Could you check a few things on this model? Use its own coordinates, in mm. A direction names the side the tool comes from. Coordinates: 2 decimals unless noted, no trailing zeros. Answer as CSV lines item,"result". Start each with the question number.
Item 1: We'd pull the mould along Y, two halves only. Please class faces 4 (the flat face through (-12, 9.525, -150)), 5 (the flat face through (12, -9.525, -150)), 6 (the cylindrical face through (15.874, -2.176, -150.266)): +Y half, -Y half, draft (parallel to the pull), parting line (faces both ways), or undercut.
Item 2: On a 3-axis mill with a long thin cutter (end or side, diameter ignored), from which of +Z, -Z, +X, -X, +Y, -Y can I reach the whole of each face in a straight line? I mean faces 1 (the flat face through (19.05, 0, -150)), 2 (the flat face through (11.892, 5, -150)), 3 (the flat face through (0, -2.667, -150)). Say none if no direction works.
Item 3: Suppose I cut it at A-A, the plane z = -233.5. State how many separate pieces and enclosed holes the cut face has, and give its area (3 significant figures).
Item 4: I'm going to push a flat-ended pin straight in: P1, Ø1, axis at y = 7.5, z = -153.5, coming from the +X side. Where does the tip first touch, or does it pass through?
Item 5: If I drill on line 1 along Y through (x, z) = (12.7, -233.5) (3 decimals); line 2 along X through (y, z) = (-3.25, -45); line 3 along X through (y, z) = (3, -258.5), over which ranges is the centre line in solid material (lowest first)? Write a range as [from, to].
Autodesk Inventor part; units mm, degrees
ref_plane "YZ Plane" through (0, 0, 0) normal (1, 0, 0) x (0, 1, 0)
ref_plane "XZ Plane" through (0, 0, 0) normal (0, 1, 0) x (-1, 0, 0)
ref_plane "XY Plane" through (0, 0, 0) normal (0, 0, 1) x (1, 0, 0)
sketch "Sketch1" plane through (0, 0, 0) normal (0, 0, 1) x (1, 0, 0)
  circle A0 centre (12.7, -3.175) radius 3.3274
  arc A1 (-12.1461, 2.3151) -> (-11.8921, 2.5691) centre (-12.1461, 2.5691) ccw
  line L0 (-17.0229, 2.3151) -> (-12.1461, 2.3151)
  arc A2 (-17.2769, 2.5691) -> (-17.0229, 2.3151) centre (-17.0229, 2.5691) ccw
  line L1 (-17.2769, 4.9059) -> (-17.2769, 2.5691)
  arc A3 (-14.4829, 7.6999) -> (-17.2769, 4.9059) centre (-14.4829, 4.9059) ccw
  line L2 (-12.1461, 7.6999) -> (-14.4829, 7.6999)
  arc A4 (-11.8921, 7.4459) -> (-12.1461, 7.6999) centre (-12.1461, 7.4459) ccw
  line L3 (-11.8921, 2.5691) -> (-11.8921, 7.4459)
  circle A5 centre (-12.7, -3.175) radius 3.3274
  arc A6 (12.1461, 7.6999) -> (11.8921, 7.4459) centre (12.1461, 7.4459) ccw
  line L4 (14.4829, 7.6999) -> (12.1461, 7.6999)
  arc A7 (17.2769, 4.9059) -> (14.4829, 7.6999) centre (14.4829, 4.9059) ccw
  line L5 (17.2769, 2.5691) -> (17.2769, 4.9059)
  arc A8 (17.0229, 2.3151) -> (17.2769, 2.5691) centre (17.0229, 2.5691) ccw
  line L6 (12.1461, 2.3151) -> (17.0229, 2.3151)
  arc A9 (11.8921, 2.5691) -> (12.1461, 2.3151) centre (12.1461, 2.5691) ccw
  line L7 (11.8921, 7.4459) -> (11.8921, 2.5691)
  line L8 (-9.4427, 9.525) -> (-14.0829, 9.525)
  arc A10 (-15.6028, 9.525) -> (-14.0829, 9.525) centre (-14.8428, 9.525) ccw
  line L9 (-15.6028, 9.525) -> (-15.875, 9.525)
  arc A11 (-15.875, 9.525) -> (-19.05, 6.35) centre (-15.875, 6.35) ccw
  line L10 (-19.05, 6.35) -> (-19.05, -6.35)
  arc A12 (-19.05, -6.35) -> (-15.875, -9.525) centre (-15.875, -6.35) ccw
  line L11 (-15.875, -9.525) -> (-15.6028, -9.525)
  arc A13 (-14.0829, -9.525) -> (-15.6028, -9.525) centre (-14.8428, -9.525) ccw
  line L12 (-14.0829, -9.525) -> (-9.4578, -9.525)
  arc A14 (-7.9379, -9.525) -> (-9.4578, -9.525) centre (-8.6979, -9.525) ccw
  line L13 (-7.9379, -9.525) -> (7.9379, -9.525)
  arc A15 (9.4578, -9.525) -> (7.9379, -9.525) centre (8.6979, -9.525) ccw
  line L14 (9.4578, -9.525) -> (14.0829, -9.525)
  arc A16 (15.6028, -9.525) -> (14.0829, -9.525) centre (14.8428, -9.525) ccw
  line L15 (15.6028, -9.525) -> (15.875, -9.525)
  arc A17 (15.875, -9.525) -> (19.05, -6.35) centre (15.875, -6.35) ccw
  line L16 (19.05, -6.35) -> (19.05, 6.35)
  arc A18 (19.05, 6.35) -> (15.875, 9.525) centre (15.875, 6.35) ccw
  line L17 (15.875, 9.525) -> (15.6028, 9.525)
  arc A19 (14.0829, 9.525) -> (15.6028, 9.525) centre (14.8428, 9.525) ccw
  line L18 (14.0829, 9.525) -> (9.4427, 9.525)
  arc A20 (7.9228, 9.525) -> (9.4427, 9.525) centre (8.6828, 9.525) ccw
  line L19 (7.9228, 9.525) -> (5.6388, 9.525)
  arc A21 (5.6388, 9.525) -> (4.064, 7.9502) centre (5.6388, 7.9502) ccw
  line L20 (4.064, 7.9502) -> (4.064, 7.0358)
  arc A22 (4.064, 7.0358) -> (5.6388, 5.461) centre (5.6388, 7.0358) ccw
  line L21 (5.6388, 5.461) -> (6.6706, 5.461)
  arc A23 (6.6706, 5.461) -> (6.9246, 5.715) centre (6.6706, 5.715) ccw
  line L22 (6.9246, 5.715) -> (6.9246, 6.081)
  arc A24 (7.1786, 6.335) -> (6.9246, 6.081) centre (7.1786, 6.081) ccw
  line L23 (7.1786, 6.335) -> (9.017, 6.335)
  arc A25 (10.287, 5.065) -> (9.017, 6.335) centre (9.017, 5.065) ccw
  line L24 (10.287, 5.065) -> (10.287, 3.6128)
  arc A26 (10.0266, 2.9842) -> (10.287, 3.6128) centre (9.398, 3.6128) ccw
  line L25 (10.0266, 2.9842) -> (5.6159, -1.4264)
  arc A27 (2.621, -2.667) -> (5.6159, -1.4264) centre (2.621, 1.5686) ccw
  line L26 (2.621, -2.667) -> (-2.621, -2.667)
  arc A28 (-5.6159, -1.4264) -> (-2.621, -2.667) centre (-2.621, 1.5686) ccw
  line L27 (-5.6159, -1.4264) -> (-10.0266, 2.9842)
  arc A29 (-10.287, 3.6128) -> (-10.0266, 2.9842) centre (-9.398, 3.6128) ccw
  line L28 (-10.287, 3.6128) -> (-10.287, 5.065)
  arc A30 (-9.017, 6.335) -> (-10.287, 5.065) centre (-9.017, 5.065) ccw
  line L29 (-9.017, 6.335) -> (-7.1786, 6.335)
  arc A31 (-6.9246, 6.081) -> (-7.1786, 6.335) centre (-7.1786, 6.081) ccw
  line L30 (-6.9246, 6.081) -> (-6.9246, 5.715)
  arc A32 (-6.9246, 5.715) -> (-6.6706, 5.461) centre (-6.6706, 5.715) ccw
  line L31 (-6.6706, 5.461) -> (-5.6388, 5.461)
  arc A33 (-5.6388, 5.461) -> (-4.064, 7.0358) centre (-5.6388, 7.0358) ccw
  line L32 (-4.064, 7.0358) -> (-4.064, 7.9502)
  arc A34 (-4.064, 7.9502) -> (-5.6388, 9.525) centre (-5.6388, 7.9502) ccw
  line L33 (-5.6388, 9.525) -> (-7.9228, 9.525)
  arc A35 (-9.4427, 9.525) -> (-7.9228, 9.525) centre (-8.6828, 9.525) ccw
  point P0 (0, 0)
extrude "Extrusion1" add sketch "Sketch1" against normal blind 304.8
properties part number "1534-LITE"
Ans:
1,face 4,"+Y half"
1,face 5,"-Y half"
1,face 6,"undercut"
2,face 1,"+Z, -Z, +X, +Y, -Y"
2,face 2,"+Z, -Z"
2,face 3,"+Z, -Z, +Y"
3,separate pieces,"1"
3,enclosed holes,"4"
3,area,"414 mm^2"
4,P1,"stops at x = 18.98"
5,line 1,"y = [-9.525, -6.502], [0.152, 2.315], [7.7, 9.525]"
5,line 2,"x = [-19.05, -16.03], [-9.37, 9.37], [16.03, 19.05]"
5,line 3,"x = [-19.05, -17.28], [-11.89, -10.04], [10.04, 11.89], [17.28, 19.05]"
